Geometry: final body of the model. Coordinates: model frame, mm. Give positions to 0.01 mm unless a question says otherwise; leave off trailing zeros. Order: outer loops, then holes, each group sorted by start corner. A loop starts at its lowest first (then second) coordinate and runs counter-clockwise, first axis right, second up. Notation, with made-up numbers: (57.25, 1.25) - (93.25, 1.25) arc R16 ccw to (93.25, 6.25) - close; hole circle Ø2 at (62, -21.75). An arc over 180 degrees is marked (long way). One line per question, with ' | ' between items. Start each with the question number.
Solid Edge part; units mm, degrees
sketch "Sketch1" plane through (0, 0, 0) normal (1, 0, 0) x (0, 1, 0)
  line L0 (-34.4456, 14.5486) -> (0, 14.5486)
  line L1 (0, 14.5486) -> (0, -15.4514)
  line L2 (-34.4456, -15.4514) -> (0, -15.4514)
  arc A0 (-34.4456, 14.5486) -> (-34.4456, -15.4514) centre (-34.4456, -0.4514) ccw
extrude "Protrusion1" add sketch "Sketch1" along normal blind 10
sketch "Sketch2" plane through (0, 0, 0) normal (1, 0, 0) x (0, 1, 0)
  circle A0 centre (-34.4456, -0.4514) radius 4.7659
extrude "Cutout1" cut sketch "Sketch2" along normal blind 53.975
(1) Cut plane D-D, the plane z = 9.25. Return the cut outline in (x, y).
(2) Contact query for flat-ended pins moving along their axis: P1, Ø6, axis at x = 5.5, z = -6, coming from the -Y side; P2, Ø6, axis at y = -25.5, z = 9.5, coming from the -X side; P3, Ø8.5, axis at y = -34.45, z = -0.45, coming from the +X side; P4, Ø4, axis at x = 7, z = 11, coming from the -Y side. Output: stop coordinate, or through.
(3) Pull-direction query (Y, two-part tool) for faces 1 (the flat face through (10, -25, 0)), 2 (the cylindrical face through (4.93, -39.207, -0.661)), 3 (the cylindrical face through (4.93, -49.44, -0.78)); classes: +Y half, -Y half, draft (parallel to the pull), parting line (faces both ways), or undercut.
(4) Cut plane A-A, the plane z = -4. Return the cut outline in (x, y).
(5) Cut plane C-C, the plane x = 1.75. Return the cut outline in (y, z).
(6) Cut plane B-B, the plane y = -37.5. Return the cut outline in (x, z).
(7) Material intervals for line 1 along Y through (x, z) = (2.25, 1.75); line 2 along Y through (x, z) = (5, -2.5); line 3 along Y through (x, z) = (3.75, -7.25), sorted ascending. Write a range as from..to.
Results are:
1) outline: (0, -45.89) - (10, -45.89) - (10, 0) - (0, 0) - close
2) P1: y = -49.23 | P2: x = 0 | P3: through | P4: y = -46.09
3) face 1: draft | face 2: undercut | face 3: -Y half
4) outline: (0, -49.02) - (10, -49.02) - (10, -37.63) - (0, -37.63) - close; (0, -31.26) - (10, -31.26) - (10, 0) - (0, 0) - close
5) outline: (-34.45, -15.45) - (0, -15.45) - (0, 14.55) - (-34.45, 14.55) arc R15 ccw to start; hole circle Ø9.53 at (-34.45, -0.45)
6) outline: (0, -15.14) - (10, -15.14) - (10, -4.11) - (0, -4.11) - close; (0, 3.21) - (10, 3.21) - (10, 14.23) - (0, 14.23) - close
7) line 1: -49.28..-38.67, -30.22..0 | line 2: -49.31..-38.75, -30.14..0 | line 3: -47.82..0
